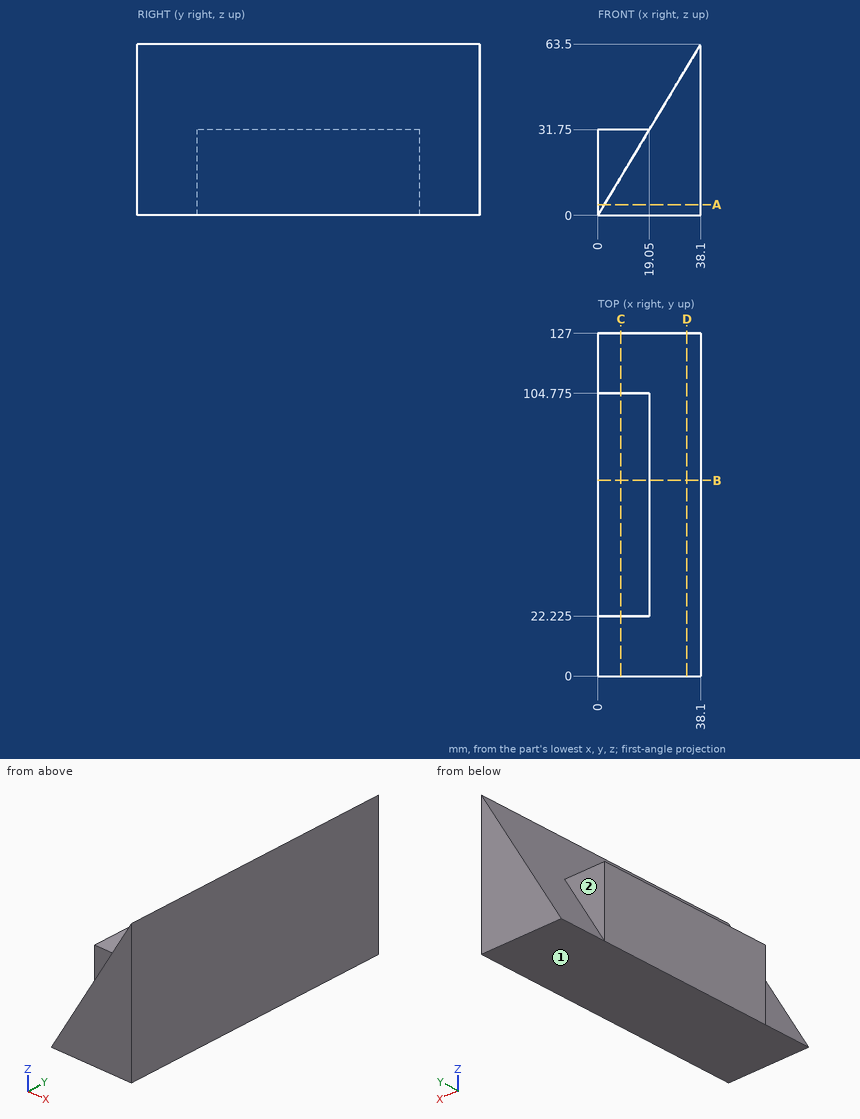
Design review of the part shown in the three views and the two pictorial views. Dimensions are in mm from the part's minimum x, y and z. A direction names the side the tool comes from. Round coordinates to 2 decimals unless told otherwise and drop trailing zeros. Write each loop counter-clockwise with the first axis right and the second up, starting at its lowest first coordinate (ties: lowest second). Pieces come first, ordered by that corner, then holes. Notation, with made-up numbers: (-0.75, 43.5) -> (5.25, 43.5) arc R18 cw to (5.25, 76.5) -> close; hole circle Ø8 at (-0.75, -37.5). An arc over 180 degrees is marked (long way). Write item = value, one per line. Start each with the question number.
1) Tool access review of the marked faces 1 and 2: name each direction out of +Z, -Z, +X, -X, +Y, -Y from which nothing blocks a thin tool from reaching the whole face with its end or side.
2) Take a section at A-A, the plane z = 4. State the section outline as (x, y) points (3 decimals).
3) Take a section at D-D, the plane x = 33. State the section outline as (y, z) points, plus the area to 4 significant figures.
4) Take a section at B-B, the plane y = 72.5. State the section outline as (x, z) points, plus the area to 3 significant figures.
5) Wall thickness on probe 1 along X at (y, z) = (34, 37); probe 2 along Z at (x, y) = (9, 28.5); probe 3 along Z at (x, y) = (32.5, 29): over which ranges is each line inside the solid? List them lowest first. Write a range as from..to.
6) Take a section at C-C, the plane x = 8.5. State the section outline as (y, z) points (3 decimals), plus the area to 3 significant figures.
7) Clearance check with flat-ended pins moving along their axes: pin 1 (6 mm diameter, centred on y = 101.5, z = 44, fed in from -X); pin 2 (3 mm diameter, centred on x = 30.5, y = 34.5, fed in from +Z); pin 3 (9.5 mm diameter, centred on x = 9, y = 76, fed in from +Z). State where each tip first meets the part, or that it passes through.
Results list:
q1.face_1 = -Z, +X, -X, +Y, -Y
q1.face_2 = +Z, -X, +Y
q2.outline = (0, 22.225) -> (2.4, 22.225) -> (2.4, 0) -> (38.1, 0) -> (38.1, 127) -> (2.4, 127) -> (2.4, 104.775) -> (0, 104.775) -> close
q3.outline = (0, 0) -> (127, 0) -> (127, 55) -> (0, 55) -> close
q3.area = 6,985 mm²
q4.outline = (0, 0) -> (38.1, 0) -> (38.1, 63.5) -> (19.05, 31.75) -> (0, 31.75) -> close
q4.area = 1,510 mm²
q5.probe_1 = 22.2..38.1
q5.probe_2 = 0..31.75
q5.probe_3 = 0..54.17
q6.outline = (0, 0) -> (127, 0) -> (127, 14.167) -> (104.775, 14.167) -> (104.775, 31.75) -> (22.225, 31.75) -> (22.225, 14.167) -> (0, 14.167) -> close
q6.area = 3,250 mm²
q7.pin_1 = 24.6
q7.pin_2 = 53.33
q7.pin_3 = 31.75
